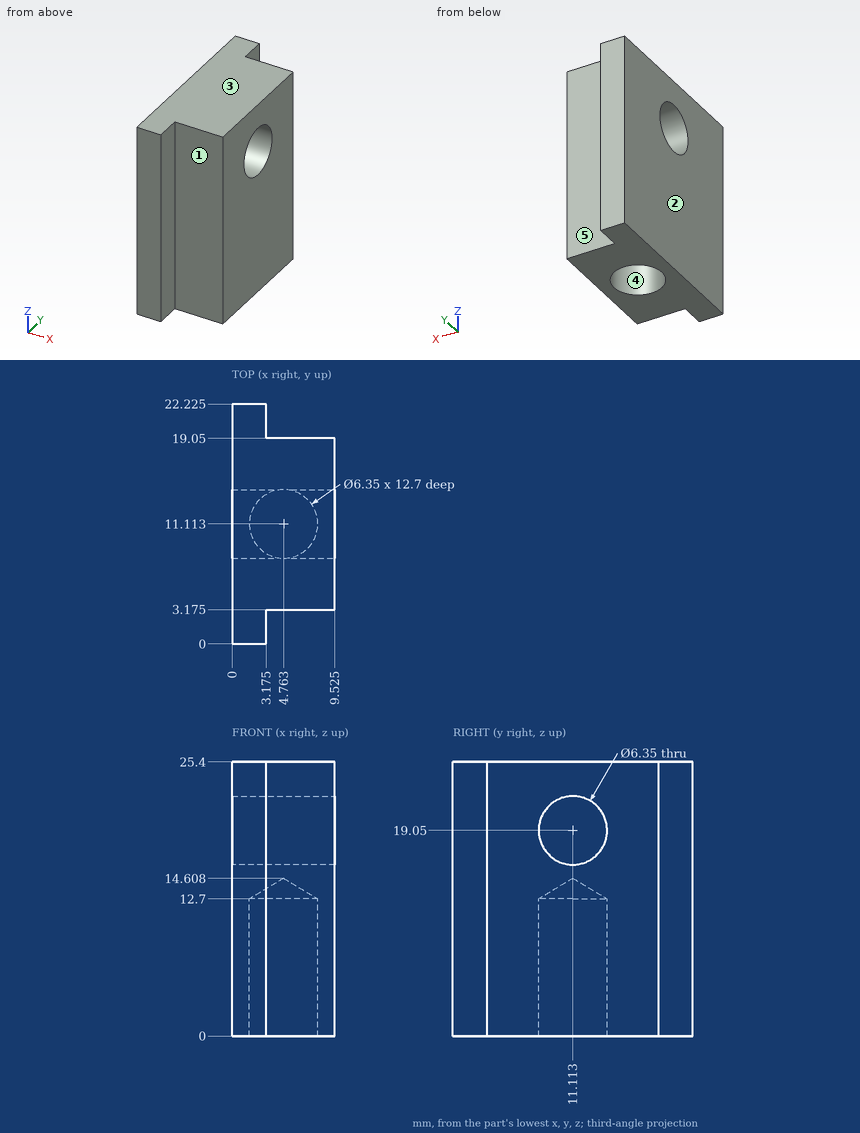
The figure shows three views and two pictorial views of one solid part (mm, origin at its lowest corner). Answer the questions. A direction names the side the tool comes from. Coordinates: 2 decimals unless noted, no trailing zeros.
(1) A tool of negligible diameter and unlimited length cuts with its end or side. For the marked faces 1 and 2, from which of +Z, -Z, +X, -X, +Y, -Y can it reach the whole face along a straight path? Write none if from no direction.
Solution:
face 1: +Z, -Z, +X, -Y
face 2: +Z, -Z, -X, +Y, -Y
(2) The mould has two halves that part along Y. Classify the marked faces 3, 4 and 5: released by +Y, released by -Y, zero draft, split by the parting line, or undercut.
Solution:
face 3: zero draft
face 4: undercut
face 5: released by +Y
(3) Flat-ended cylindrical pins translate along their axes: pin 1 Ø1.5 at (x, z) = (8, 4.5) entering from +Y; pin 2 Ø1.6 at (y, z) = (20.5, 11.5) entering from +X (1 decimal). Find the tip coordinate at first contact, or state that the pin passes through.
Solution:
pin 1: stops at y = 19.05
pin 2: stops at x = 3.2
(4) Consider line 1 along X through (y, z) = (11.5, 4.75) (1 decimal); line 2 along X through (y, z) = (20.75, 6) (1 decimal); line 3 along Z through (x, y) = (8.75, 13) (1 decimal). Determine where each line is inside the solid, lowest interval first.
Solution:
line 1: x = 0 to 1.6, 7.9 to 9.5
line 2: x = 0 to 3.2
line 3: z = 0 to 16.5, 21.6 to 25.4
